Verification items for the finished model (mm, model axes). Face numbers are marked on the shaded views. A direction names the side the tool comes from. Give positions to 0.01 mm unless a question says otherwise; leave off trailing zeros. Loops run counter-clockwise (first coordinate to the right, second up) from the corner with the lowest first, then second, coordinate; pieces in that order, holes last. Notation, with made-up numbers: (42, 67) - (88, 67) arc R13 ccw to (88, 73) - close; hole circle Ø6 at (37.5, -7). An arc over 180 degrees is marked (long way). One line per question, with ' | ' between items. Start each with the question number.
1. Mould release check, pull along X, two halves, no side actions. Record for the marked faces 1, 2 and 3: +X half, -X half, draft (parallel to the pull), parting line (faces both ways), or undercut.
2. Section check B-B, the plane y = 6.25. Enter the section's corners in (x, z), then the cut area to 3 significant figures.
3. Tool access check on the marked faces 4, 5 and 6. Record the directions out of +Z, -Z, +X, -X, +Y, -Y that give a thin tool (end or side, any length) a straight path to the whole face; none if there is none.
4. Section check D-D, the plane z = 16.5. Enter the section's corners in (x, y).
5. Thickness scan on line 1 along X through (y, z) = (5, 5); line 2 along X through (y, z) = (5.25, -5.5); line 3 along Z through (x, y) = (0, 1.75). Record the ranges inside material, lowest first. Write a range as from..to.
6. Section check C-C, the plane x = -11. Enter the section's corners in (y, z).
7. Depth check by flat-ended pin: pin 1 Ø1.5 at (y, z) = (2, 1) entering from +X; pin 2 Ø5.5 at (x, z) = (5.48, 5.48) entering from +Y; pin 3 Ø4 at (x, z) = (-5.48, 5.48) entering from -Y; pin 4 Ø4 at (x, y) = (-8.5, 12) entering from +Z. Enter the tip coordinate at first touch or a pass-through.
8. Section check A-A, the plane x = 0. Enter the section's corners in (y, z), then the cut area to 3 significant figures.
from build123d import *

# Parameters (mm, degrees)
SKETCH1_R      = 20.05
SKETCH1_R_2    = 3.25
SKETCH1_R_3    = 1.75
EXTRUDE1_DEPTH = 15
SKETCH7_R      = 3.15
EXTRUDE4_DEPTH = 3.5
SKETCH8_R      = 20.05
SKETCH8_R_2    = 12.5
EXTRUDE5_DEPTH = 11


with BuildPart() as part:
    # Sketch1 → Extrude1 (new body)
    with BuildSketch(Plane(origin=(0, 0, 0), x_dir=(1, 0, 0), z_dir=(0, 1, 0))):
        Circle(SKETCH1_R)
        Circle(SKETCH1_R_2, mode=Mode.SUBTRACT)
        with Locations((5.480077554, 5.480077554)):
            Circle(SKETCH1_R_3, mode=Mode.SUBTRACT)
        with Locations((5.480077554, -5.480077554)):
            Circle(SKETCH1_R_3, mode=Mode.SUBTRACT)
        with Locations((-5.480077554, -5.480077554)):
            Circle(SKETCH1_R_3, mode=Mode.SUBTRACT)
        with Locations((-5.480077554, 5.480077554)):
            Circle(SKETCH1_R_3, mode=Mode.SUBTRACT)
        with Locations((-10.044563579, -13.090330115)):
            Circle(SKETCH1_R_3, mode=Mode.SUBTRACT)
        with Locations((-6.314276634, 15.244012286)):
            Circle(SKETCH1_R_3, mode=Mode.SUBTRACT)
        with Locations((16.358840213, -2.153682172)):
            Circle(SKETCH1_R_3, mode=Mode.SUBTRACT)
    extrude(amount=EXTRUDE1_DEPTH)

    # Sketch7 → Extrude4 (cut)
    with BuildSketch(Plane(origin=(0, 15, 0), x_dir=(1, 0, 0), z_dir=(0, 1, 0))):
        with Locations((-5.480077554, 5.480077554)):
            Circle(SKETCH7_R)
        with Locations((5.480077554, 5.480077554)):
            Circle(SKETCH7_R)
        with Locations((5.480077554, -5.480077554)):
            Circle(SKETCH7_R)
        with Locations((-5.480077554, -5.480077554)):
            Circle(SKETCH7_R)
    extrude(amount=-EXTRUDE4_DEPTH, mode=Mode.SUBTRACT)

    # Sketch8 → Extrude5 (cut)
    with BuildSketch(Plane.XZ):
        Circle(SKETCH8_R)
        Circle(SKETCH8_R_2, mode=Mode.SUBTRACT)
    extrude(amount=-EXTRUDE5_DEPTH, mode=Mode.SUBTRACT)


solid = part.part
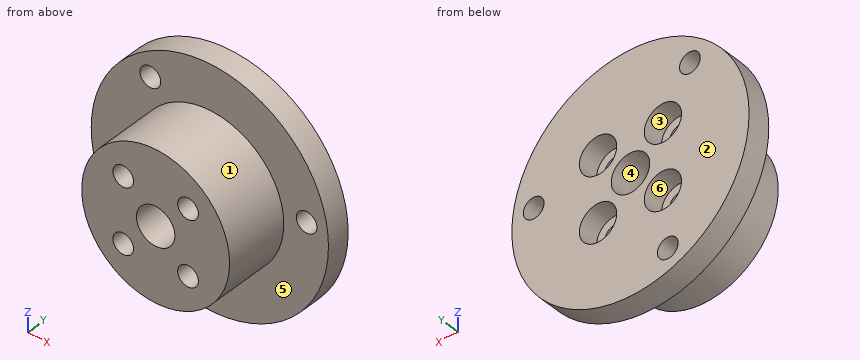
Results list:
1) face 1: parting line | face 2: draft | face 3: undercut
2) outline: circle Ø25 at (0, 0); hole circle Ø3.5 at (-5.48, -5.48); hole circle Ø3.5 at (-5.48, 5.48); hole circle Ø6.5 at (0, 0); hole circle Ø3.5 at (5.48, -5.48); hole circle Ø3.5 at (5.48, 5.48) | area: 419 mm²
3) face 4: +Y, -Y | face 5: -Y | face 6: +Y
4) outline: (-11.39, 11) - (11.39, 11) - (11.39, 15) - (-11.39, 15) - close
5) line 1: -11.46..-7.16, -3.8..3.8, 7.16..11.46 | line 2: -11.22..-7.23, -3.73..3.73, 7.23..11.22 | line 3: -12.5..-3.25, 3.25..12.5
6) outline: (0, -5.94) - (11, -5.94) - (11, -16.76) - (15, -16.76) - (15, 11.62) - (11, 11.62) - (11, 5.94) - (0, 5.94) - close; (11, 14.56) - (15, 14.56) - (15, 16.76) - (11, 16.76) - close
7) pin 1: x = 12.5 | pin 2: y = 11.5 | pin 3: y = 0 | pin 4: z = 18.97
8) outline: (0, -12.5) - (11, -12.5) - (11, -20.05) - (15, -20.05) - (15, -3.25) - (0, -3.25) - close; (0, 3.25) - (15, 3.25) - (15, 20.05) - (11, 20.05) - (11, 12.5) - (0, 12.5) - close | area: 338 mm²
